Here's how the part is built. I have some questions about the finished solid (model axes, mm). Face numbers are marked on the shaded views. A direction names the side the tool comes from. Coordinates: 2 decimals unless noted, no trailing zeros. Write each loop counter-clockwise with the first axis right and the second up, starting at its lowest first coordinate (ties: lowest second). Pieces come first, ordered by that corner, then holes.
Item 1: If we section it at C-C (y = -104): Please give me the cut outline in (x, z), then the cut area to 3 significant figures.
Item 2: I'm going to push flat-ended pins straight in: pin 1 Ø2.5 at (x, y) = (-21, 5) entering from +Z; pin 2 Ø4 at (x, z) = (-17.5, 5.5) entering from +Y; pin 3 Ø2.5 at (x, y) = (-19.8, 5) entering from -Z; pin 4 Ø4 at (y, z) = (-124, 1) entering from -X. Where does each tip first touch, or does it pass through?
Item 3: For the marked faces 1 and 2, which set-ups out of +Z, -Z, +X, -X, +Y, -Y let a thin tool reach every point of the face, with its end or its side?
Item 4: If I drill on line 1 (Y direction, x = -19.8, z = 2.4); line 2 (X direction, y = -0.5, z = 5.5); line 3 (Y direction, x = -9.5, z = 6.75), over which ranges is the centre line in solid material (lowest first)?
Item 5: If we section it at B-B (x = -19.8): Please give me the cut outline in (y, z).
Item 6: If we section it at D-D (x = -0.5): Please give me the cut outline in (y, z).
Item 7: If we section it at A-A (z = 5.75): Please give me the cut outline in (x, y).
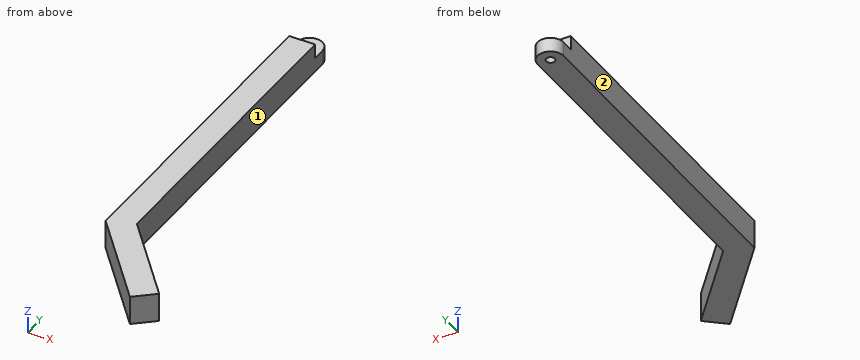
from build123d import *

# Parameters (mm, degrees)
SKETCH_4_W          = 9
SKETCH_4_H          = 10
EXTRUDE_2_DEPTH     = 10
CUT_EXTRUDE_1_DEPTH = 10
SKETCH_4_2_W        = 9
SKETCH_4_2_H        = 10
CUT_EXTRUDE_START   = 10
CUT_EXTRUDE_2_DEPTH = 10
SKETCH_8_R          = 1.5
CUT_EXTRUDE_3_DEPTH = 10


with BuildPart() as part:
    # 草图4 → 凸台-拉伸2 (new body)
    with BuildSketch(Plane(origin=(0, 0, 0), x_dir=(1, 0, 0), z_dir=(0, 1, 0))):
        with Locations((-19.8, -3.957142857)):
            Rectangle(SKETCH_4_W, SKETCH_4_H)
    extrude(amount=EXTRUDE_2_DEPTH)

    # 草图6 → 切除-拉伸1 (cut)
    with BuildSketch(Plane.XY.offset(8.957142857)):
        with BuildLine():
            Line((-24.3, 10), (-24.3, 5))
            ThreePointArc((-24.3, 5), (-19.8, 9.5), (-15.3, 5))
            Line((-15.3, 5), (-15.3, 10))
            Line((-15.3, 10), (-24.3, 10))
        make_face()
    extrude(amount=-CUT_EXTRUDE_1_DEPTH, mode=Mode.SUBTRACT)

    # 扫描2: sweep along a path in 草图5
    with BuildLine(Plane.XY.offset(3.957142857)) as sweep_2_path:
        Line((-19.8, 0), (-19.8, -110))
        Line((-19.8, -110), (5.372988935, -140))
    # 草图4<2> → 扫描2 (sweep)
    with BuildSketch(Plane(origin=(0, 0, 0), x_dir=(1, 0, 0), z_dir=(0, 1, 0))):
        with Locations((-19.8, -3.957142857)):
            Rectangle(SKETCH_4_2_W, SKETCH_4_2_H)
    sweep(path=sweep_2_path.line, transition=Transition.RIGHT)

    # 草图7 → 切除-拉伸2 (cut)
    with BuildSketch(Plane.XY.offset(3.957142857).offset(CUT_EXTRUDE_START)):
        with BuildLine():
            Line((-24.3, 5), (-24.3, 0.5))
            Line((-24.3, 0.5), (-15.3, 0.5))
            Line((-15.3, 0.5), (-15.3, 5))
            ThreePointArc((-15.3, 5), (-19.8, 9.5), (-24.3, 5))
        make_face()
    extrude(amount=-CUT_EXTRUDE_2_DEPTH, mode=Mode.SUBTRACT)

    # 草图8 → 切除-拉伸3 (cut)
    with BuildSketch(Plane.XY.offset(3.957142857)):
        with Locations((-19.8, 5)):
            Circle(SKETCH_8_R)
    extrude(amount=-CUT_EXTRUDE_3_DEPTH, mode=Mode.SUBTRACT)


solid = part.part
Answer list:
1. outline: (-24.3, -1.04) - (-15.3, -1.04) - (-15.3, 8.96) - (-24.3, 8.96) - close
1. area: 90.0 mm2
2. pin 1: stops at z = 3.96
2. pin 2: stops at y = 9.38
2. pin 3: passes through
2. pin 4: stops at x = -15.61
3. face 1: +Z, -Z, +X, +Y
3. face 2: +Z, -Z, -X, +Y, -Y
4. line 1: y = -117 to 3.5, 6.5 to 9.5
4. line 2: x = -24.3 to -15.3
4. line 3: y = -129.28 to -115.27
5. outline: (-117, -1.04) - (3.5, -1.04) - (3.5, 3.96) - (0.5, 3.96) - (0.5, 8.96) - (-117, 8.96) - close; (6.5, -1.04) - (9.5, -1.04) - (9.5, 3.96) - (6.5, 3.96) - close
6. outline: (-140, -1.04) - (-126, -1.04) - (-126, 8.96) - (-140, 8.96) - close
7. outline: (-24.3, -111.64) - (1.93, -142.89) - (8.82, -137.11) - (-15.3, -108.36) - (-15.3, 0.5) - (-24.3, 0.5) - close
